```python
from build123d import *

# Parameters (mm, degrees)
F0_W     = 111.186231
F0_H     = 64.043274
F0_R     = 16.170621
F1_DEPTH = 199.644
F2_SIZE  = 5.08
F3_W     = 101.026231
F3_H     = 53.883274
F3_R     = 21.250621
F4_DEPTH = 127


with BuildPart() as f1:
    # F0 (on Front) → F1 (new body)
    with BuildSketch(Plane.XZ):
        with Locations((-73.523032, -39.80646)):
            Rectangle(F0_W, F0_H)
        with Locations((-101.097219, -35.803754)):
            Circle(F0_R, mode=Mode.SUBTRACT)
    extrude(amount=F1_DEPTH)

    # F2
    f2_edges = [f1.edges().sort_by_distance(p)[0] for p in [
        (-73.523032, -199.644, -7.784823),
        (-129.116148, -199.644, -39.80646),
        (-73.523032, -199.644, -71.828097),
        (-17.929917, -199.644, -39.80646),
        (-117.26784, -199.644, -35.803754),
    ]]
    chamfer(f2_edges, length=F2_SIZE)

    # F3 (on face) → F4 (join)
    with BuildSketch(Plane.XZ.offset(199.644)):
        with BuildLine():
            ThreePointArc((-62.805545, -55.70646), (-63.026238, -55.425729), (-63.238576, -55.138626))
            Line((-63.238576, -55.138626), (-63.238576, -55.70646))
            Line((-63.238576, -55.70646), (-62.805545, -55.70646))
        make_face()
        with BuildLine():
            ThreePointArc((-62.805545, -55.70646), (-53.377099, -60.202052), (-43.948654, -55.70646))
            Line((-43.948654, -55.70646), (-62.805545, -55.70646))
        make_face()
        with Locations((-73.523032, -39.80646)):
            Rectangle(F3_W, F3_H)
        with BuildLine():
            Line((-63.238576, -40.99594), (-63.238576, -25.149755))
            Line((-63.238576, -25.149755), (-40.182158, -25.149755))
            Line((-40.182158, -25.149755), (-40.182158, -55.70646))
            Line((-40.182158, -55.70646), (-43.948654, -55.70646))
            ThreePointArc((-43.948654, -55.70646), (-53.377099, -60.202052), (-62.805545, -55.70646))
            Line((-62.805545, -55.70646), (-63.238576, -55.70646))
            Line((-63.238576, -55.70646), (-63.238576, -55.138626))
            ThreePointArc((-63.238576, -55.138626), (-65.511868, -48.067283), (-63.238576, -40.99594))
        make_face(mode=Mode.SUBTRACT)
        with Locations((-101.097219, -35.803754)):
            Circle(F3_R, mode=Mode.SUBTRACT)
        with BuildLine():
            Line((-40.182158, -25.149755), (-63.238576, -25.149755))
            Line((-63.238576, -25.149755), (-63.238576, -40.99594))
            Line((-63.238576, -40.99594), (-63.238576, -55.138626))
            ThreePointArc((-63.238576, -55.138626), (-63.026238, -55.425729), (-62.805545, -55.70646))
            Line((-62.805545, -55.70646), (-43.948654, -55.70646))
            Line((-43.948654, -55.70646), (-40.182158, -55.70646))
            Line((-40.182158, -55.70646), (-40.182158, -25.149755))
        make_face()
    extrude(amount=-F4_DEPTH)


solid = f1.part
```
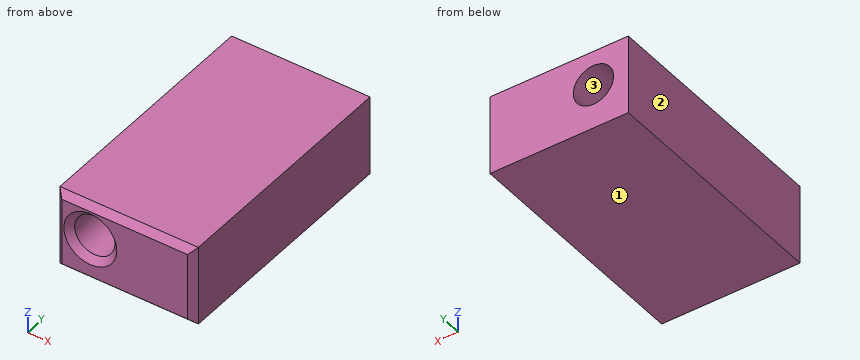
The model under review builds one solid part; all positions refer to its coordinate system, in mm. Face numbers are marked on the shaded views. Give positions to 0.01 mm unless a question says otherwise; leave off trailing zeros. Loops run counter-clockwise (first coordinate to the right, second up) from the corner with the lowest first, then second, coordinate; pieces in that order, holes last. Notation, with made-up numbers: (-7.75, 77.5) - (16.25, 77.5) arc R14 cw to (16.25, 99.5) - close; hole circle Ø8 at (57.25, 77.25). An arc over 180 degrees is marked (long way). Answer as a JSON object with one key per item and string values.
Q1. To check wall thickness, follow line 1 along X through (y, z) = (-107.5, -37); line 2 along Z through (x, y) = (-101, -113.5); line 3 along X through (y, z) = (-85, -35.5). State the ranges of each line that lie inside material, in increasing order.
Worked out:
{"line 1": "x = -129.12 to -117.22, -84.97 to -17.93", "line 2": "z = -71.83 to -51.97, -19.63 to -7.78", "line 3": "x = -129.12 to -117.26, -84.93 to -17.93"}
Q2. Mouldability with a two-part tool opening along Z and no side actions: class the marked faces 1, 2 and 3 as +Z half, -Z half, draft (parallel to the pull), parting line (faces both ways), or undercut.
Worked out:
{"face 1": "-Z half", "face 2": "draft", "face 3": "undercut"}
Q3. Add section A-A on y = -22.5. State the section outline as (x, z) points, plus the area to 3 significant figures.
Worked out:
{"outline": "(-129.12, -71.83) - (-17.93, -71.83) - (-17.93, -7.78) - (-129.12, -7.78) - close; hole circle Ø32.34 at (-101.1, -35.8)", "area": "6,300 mm^2"}
